```python
from build123d import *

# Parameters (mm, degrees)
F1_DEPTH = 101.6
F3_DEPTH = 78.232
F5_DEPTH = 32.512


with BuildPart() as f1:
    # F0 (on Front) → F1 (new body, symmetric)
    with BuildSketch(Plane.XZ):
        Polygon((0, 25.4), (0, 0), (127, 0), (177.8, 50.8), (228.6, 0), (255.540768, 26.940768), (204.740768, 77.740768), (179.340768, 103.140768), (128.540768, 153.940768), (101.6, 127), (152.4, 76.2), (101.6, 25.4), align=None)
    extrude(amount=F1_DEPTH, both=True)

    # F2 (on face) → F3 (cut)
    with BuildSketch(Plane(origin=(141.240768, 0, 141.240768), x_dir=(0.707107, 0, -0.707107), z_dir=(0.707107, 0, 0.707107))):
        with BuildLine():
            Line((-5.260512, 50.8), (-5.260512, -50.8))
            ThreePointArc((-5.260512, -50.8), (20.139488, -76.2), (45.539488, -50.8))
            Line((45.539488, -50.8), (45.539488, 50.8))
            ThreePointArc((45.539488, 50.8), (20.139488, 76.2), (-5.260512, 50.8))
        make_face()
        with BuildLine():
            Line((96.339488, 50.8), (96.339488, -50.8))
            ThreePointArc((96.339488, -50.8), (121.610302, -76.199671), (147.138174, -51.058367))
            Line((147.138174, -51.058367), (147.138174, -50.541633))
            Line((147.138174, -50.541633), (147.138174, 50.541633))
            ThreePointArc((147.138174, 50.541633), (121.868673, 76.199671), (96.339488, 50.8))
        make_face()
    extrude(amount=-F3_DEPTH, mode=Mode.SUBTRACT)

    # F4 (on face) → F5 (cut)
    with BuildSketch(Plane.XY.offset(25.4)):
        with BuildLine():
            Line((50.8, 25.4), (0, 25.4))
            Line((0, 25.4), (0, -25.4))
            Line((0, -25.4), (50.8, -25.4))
            ThreePointArc((50.8, -25.4), (76.2, 0), (50.8, 25.4))
        make_face()
    extrude(amount=-F5_DEPTH, mode=Mode.SUBTRACT)


solid = f1.part
```
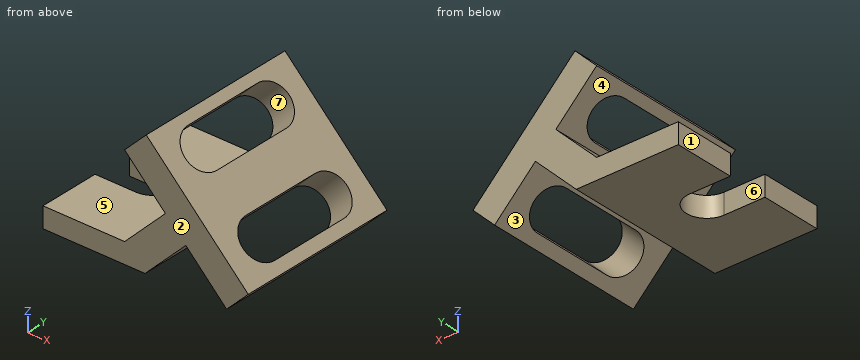
Geometry check sheet. Reference: the model listing, model coordinates, mm. Face numbers are marked on the shaded views. A direction names the side the tool comes from. Give positions to 0.01 mm unless a question says otherwise; leave off trailing zeros. Loops run counter-clockwise (first coordinate to the right, second up) from the corner with the lowest first, then second, coordinate; pieces in that order, holes last. Notation, with made-up numbers: (40, 81.25) - (82, 81.25) arc R18 ccw to (82, 85.25) - close; hole circle Ø2 at (-9, 50.5). An arc over 180 degrees is marked (long way). Use CSV: the item, a comma, the result in double quotes. Start each with the question number.
Q1. Section check B-B, the plane y = 14.5. Record the cut outline in (x, z), and give its area (3 significant figures).
Q2. Scan lines: probe 1 along Z at (x, y) = (114.5, -26); probe 2 along X at (y, z) = (-10, 15); probe 3 along X at (y, z) = (-34, 31). Record each from-to range of solid material in increasing order. Write a range as from..to.
Q3. Go/stop test with flat-tipped pins: pin 1 Ø6 at (y, z) = (9, 68.5) entering from -X; pin 2 Ø3 at (x, y) = (195, 45.5) entering from -Z; pin 3 Ø1.5 at (x, y) = (40.5, 49.5) entering from +Z. Record where each tip stops, or that it passes through.
Q4. Release check for a two-part mould opening along X. For the marked faces 1, 2 and 3 record: +X half, -X half, draft (parallel to the pull), parting line (faces both ways), or undercut.
Q5. Access from +Z, -Z, +X, -X, +Y, -Y to the whole of each face (thin tool, end or side, straight path). Record for the marked faces 4, 5, 6 and 7.
Q6. Section check C-C, the plane x = 95. Record the cut outline in (y, z), and give its area (3 significant figures).
Q7. Section check A-A, the plane y = -37. Record the cut outline in (x, z), and give its area (3 significant figures).
Findings below:
1,outline,"(71.65, 0) - (127, 0) - (177.8, 50.8) - (182.42, 46.18) - (209.36, 73.12) - (173.44, 109.04) - (146.5, 82.1) - (152.4, 76.2) - (101.6, 25.4) - (71.65, 25.4) - close; (101.6, 127) - (110.58, 118.02) - (137.52, 144.96) - (128.54, 153.94) - close; (218.34, 10.26) - (228.6, 0) - (255.54, 26.94) - (245.28, 37.2) - close"
1,area,"6,640 mm^2"
2,probe 1,"z = 0..38.3, 121.94..139.9"
2,probe 2,"x = 74.15..142, 223.08..243.6"
2,probe 3,"x = 107.2..158, 239.08..251.48"
3,pin 1,"stops at x = 141.7"
3,pin 2,"stops at z = 57.26"
3,pin 3,"stops at z = 25.4"
4,face 1,"-X half"
4,face 2,"draft"
4,face 3,"undercut"
5,face 4,"-X, +Y, -Y"
5,face 5,"+Z, -X, +Y, -Y"
5,face 6,"+Z, -Z, -X"
5,face 7,"none"
6,outline,"(-101.6, 0) - (101.6, 0) - (101.6, 25.4) - (-101.6, 25.4) - close"
6,area,"5,160 mm^2"
7,outline,"(0, 0) - (127, 0) - (177.8, 50.8) - (182.42, 46.18) - (209.36, 73.12) - (173.44, 109.04) - (146.5, 82.1) - (152.4, 76.2) - (101.6, 25.4) - (0, 25.4) - close; (101.6, 127) - (110.58, 118.02) - (137.52, 144.96) - (128.54, 153.94) - close; (218.34, 10.26) - (228.6, 0) - (255.54, 26.94) - (245.28, 37.2) - close"
7,area,"8,460 mm^2"
